from build123d import *

# Parameters (mm, degrees)
F4_DEPTH = 27.5
F5_DEPTH = 27
F6_DEPTH = 25
F7_SIZE  = 1
F8_SIZE  = 0.49999


# Not quite as in the source:
# - a fillet or chamfer is up to 0.001 mm smaller than in the source, because OpenCascade refuses the exact size


with BuildPart() as f4:
    # F3 (on Right) → F4 (new body, symmetric)
    with BuildSketch(Plane.YZ):
        Polygon((-75, 2), (-77, 2), (-79, 2), (-79, 0), (-77, 0), (0, 0), (77, 0), (79, 0), (79, 2), (77, 2), (75, 2), (60, 2), (0, 2), (-60, 2), align=None)
    extrude(amount=F4_DEPTH, both=True)

    # F3 (on Right) → F5 (join, symmetric)
    with BuildSketch(Plane.YZ):
        Polygon((-75, 32), (-77, 32), (-77, 2), (-75, 2), (-75, 17), align=None)
        Polygon((75, 32), (75, 17), (75, 2), (77, 2), (77, 32), align=None)
        Polygon((-75, 17), (-75, 2), (-60, 2), align=None)
        Polygon((75, 17), (60, 2), (75, 2), align=None)
    extrude(amount=F5_DEPTH, both=True)

    # F3 (on Right) → F6 (cut, symmetric)
    with BuildSketch(Plane.YZ):
        Polygon((-75, 17), (-75, 2), (-60, 2), align=None)
        Polygon((75, 17), (60, 2), (75, 2), align=None)
    extrude(amount=F6_DEPTH, both=True, mode=Mode.SUBTRACT)

    # F7
    f7_edges = [f4.edges().sort_by_distance(p)[0] for p in [
        (0, -75, 2),
        (0, 75, 2),
    ]]
    chamfer(f7_edges, length=F7_SIZE)

    # F8 (size 0.5 in the source; OpenCascade refuses exactly that, so slightly less here)
    f8_edges = [f4.edges().sort_by_distance(p)[0] for p in [
        (27.5, 0, 2),
        (27.5, 0, 0),
        (-27.5, 0, 2),
        (-27.5, 0, 0),
    ]]
    chamfer(f8_edges, length=F8_SIZE)


solid = f4.part
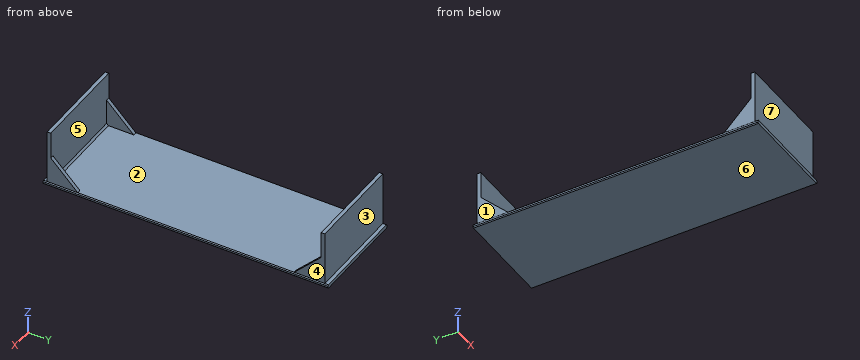
Input: part model. Units: mm. Frame: model coordinates. Face numbers are marked on the shaded views. A direction names the side the tool comes from. Give positions to 0.01 mm unless a question says otherwise; leave off trailing zeros. Order: outer loops, then holes, each group sorted by start corner. A loop starts at its lowest first (then second) coordinate and runs counter-clockwise, first axis right, second up. Notation, with made-up numbers: M 89.5,-36.75 L 148.5,-36.75 A21 ccw 148.5,-24.75 Z; hole C 19,38 d1. An arc over 180 degrees is marked long. Answer as a JSON object with one key per item and string values.
1. Cut plane C-C, the plane z = 27.5. Output: boundary loops of the cut face in (x, y), and give its area (3 significant figures).
Result sheet:
{"outline": "M -27,-77 L 27,-77 L 27,-75 L -27,-75 Z; M -27,75 L 27,75 L 27,77 L -27,77 Z", "area": "216 mm²"}
2. Cut plane A-A, the plane z = 11. Output: boundary loops of the cut face in (x, y).
Result sheet:
{"outline": "M -27,-77 L 27,-77 L 27,-69 L 25,-69 L 25,-75 L -25,-75 L -25,-69 L -27,-69 Z; M -27,69 L -25,69 L -25,75 L 25,75 L 25,69 L 27,69 L 27,77 L -27,77 Z"}
3. Cut plane B-B, the plane y = -47. Output: boundary loops of the cut face in (x, z).
Result sheet:
{"outline": "M -27.5,0.5 L -27,0 L 27,0 L 27.5,0.5 L 27.5,1.5 L 27,2 L -27,2 L -27.5,1.5 Z"}
4. Ray query, line 1 (Y direction, x = -15, z = 3); line 2 (Z direction, x = -23.5, y = 38.5); line 3 (X direction, y = -71, z = 4). Return the intervals inside material, ascending. Write a range as [from, to].
Result sheet:
{"line 1": "[-77, -75], [75, 77]", "line 2": "[0, 2]", "line 3": "[-27, -25], [25, 27]"}
5. Reachability of the marked faces 4, 5, 6 and 7 from +Z, -Z, +X, -X, +Y, -Y: full face, straight path, thin tool, end or side. Return the list, or none.
Result sheet:
{"face 4": "+Z, +X, +Y, -Y", "face 5": "+Z", "face 6": "-Z, +X, -X, +Y, -Y", "face 7": "+Z, +X, -X, -Y"}
6. Pull-direction query (Y, two-part tool) for the marked faces 1, 2 and 3; classes: +Y half, -Y half, draft (parallel to the pull), parting line (faces both ways), or undercut.
Result sheet:
{"face 1": "draft", "face 2": "undercut", "face 3": "+Y half"}
7. Cut plane D-D, the plane x = -15.5. Output: boundary loops of the cut face in (y, z).
Result sheet:
{"outline": "M -79,0 L 79,0 L 79,2 L 77,2 L 77,32 L 75,32 L 75,3 L 74,2 L -74,2 L -75,3 L -75,32 L -77,32 L -77,2 L -79,2 Z"}
8. First-contact query: P1, Ø8.5, axis at x = -13, z = 21, coming from the -Y side; P2, Ø15, axis at x = -11.5, z = 14.5, coming from the +Y side; P3, Ø6, axis at x = 3, y = -21.5, coming from the +Z side. Flat tips, straight axial feed; report the tip coordinate or a pass-through.
Result sheet:
{"P1": "y = -77", "P2": "y = 77", "P3": "z = 2"}
